Autodesk Inventor part; units mm, degrees
ref_plane "Work Plane1" through (0, 41.8, -12.9) normal (0, 0, 1) x (1, 0, 0)
ref_plane "YZ Plane" through (0, 0, 0) normal (1, 0, 0) x (0, 1, 0)
ref_plane "XZ Plane" through (0, 0, 0) normal (0, 1, 0) x (-1, 0, 0)
ref_plane "Work Plane1" through (0, 41.8, -12.9) normal (0, 0, 1) x (1, 0, 0)
sketch "Sketch1" plane through (0, 41.8, -12.9) normal (0, 0, 1) x (1, 0, 0)
  line L0 (3.85, 0.3752) -> (3.85, 4) construction
  line L1 (3.85, 4) -> (-2, 4) construction
  arc A0 (-2, 4) -> (-4, 2) centre (-2, 2) ccw construction
  line L2 (-4, 2) -> (-4, -3.85) construction
  line L3 (-4, -3.85) -> (-0.3752, -3.85) construction
  line L4 (-2, 4) -> (43.8, 4)
  line L5 (45.8, 2) -> (45.8, -43.8)
  line L6 (43.8, -45.8) -> (-2, -45.8)
  line L7 (-4, -43.8) -> (-4, 2)
  line L8 (40.3, -37.8) -> (40.3, -4)
  line L9 (37.8, -1.5) -> (4, -1.5)
  line L10 (1.5, -4) -> (1.5, -37.8)
  line L11 (4, -40.3) -> (37.8, -40.3)
  line L12 (37.8, -40.3) -> (40.3, -37.8)
  line L13 (4, -40.3) -> (1.5, -37.8)
  line L14 (4, -1.5) -> (1.5, -4)
  line L15 (40.3, -4) -> (37.8, -1.5)
  arc A1 (45.8, 2) -> (43.8, 4) centre (43.8, 2) ccw
  arc A2 (43.8, -45.8) -> (45.8, -43.8) centre (43.8, -43.8) ccw
  arc A3 (-4, -43.8) -> (-2, -45.8) centre (-2, -43.8) ccw
  arc A4 (-2, 4) -> (-4, 2) centre (-2, 2) ccw
  circle A5 centre (1, -1) radius 1.4
  circle A6 centre (40.8, -1) radius 1.4
  circle A7 centre (40.8, -40.8) radius 1.4
  circle A8 centre (1, -40.8) radius 1.4
  circle A9 centre (20.9, -20.9) radius 19.4 construction
  line L16 (3.85, -3.85) -> (3.85, -37.95)
  line L17 (3.85, -37.95) -> (37.95, -37.95)
  line L18 (37.95, -37.95) -> (37.95, -3.85)
  line L19 (37.95, -3.85) -> (3.85, -3.85)
  arc A10 (2.2654, -1.2094) -> (1.2094, -2.2654) centre (0.9, -0.9) ccw
  line L20 (2.2654, -1.2094) -> (3.85, 0.3752)
  line L21 (-0.3752, -3.85) -> (1.2094, -2.2654)
  point P0 (45.8, -45.8)
  point P1 (45.8, 4)
  point P2 (-4, -45.8)
  point P3 (40.3, -40.3)
  point P4 (40.3, -1.5)
  point P5 (1.5, -1.5)
  point P6 (1.5, -40.3)
  point P7 (40.8, -1)
  dimension "d55" = 2.8
  dimension "d34" = 49.8
  dimension "d35" = 49.8
  dimension "d36" = 5.5
  dimension "d37" = 2.5
  dimension "d38" = 2.5
  dimension "d39" = 2.5
  dimension "d40" = 2.5
  dimension "d41" = 2.5
  dimension "d42" = 2.5
  dimension "d43" = 2.5
  dimension "d44" = 2.5
  dimension "d45" = 2
  dimension "d46" = 5
  dimension "d47" = 5
  dimension "d48" = 5
  dimension "d49" = 5
  dimension "d51" = 5
  dimension "d52" = 0.5
  dimension "d53" = 5
  dimension "d54" = 5
  dimension "d56" = 2.8
  dimension "d57" = 2.8
  dimension "d58" = 2.8
  dimension "d90" = 7.85
extrude "Extrusion1" add sketch "Sketch1" along normal blind 7.7 contours L4 A1 L5 A2 L6 A3 L7 A4 | L12 L11 L13 L10 L14 L9 L15 L8 | A5 A10
fillet "Fillet1" radius 2 8 edges at (20.9, -4, -5.2) (45.2142, -3.4142, -5.2) (45.8, 20.9, -5.2) (45.2142, 45.2142, -5.2) (20.9, 45.8, -5.2) (-3.4142, 45.2142, -5.2) (-4, 20.9, -5.2) (-3.4142, -3.4142, -5.2)
sketch "Sketch3" plane through (0, 41.8, -5.2) normal (0, 0, 1) x (1, 0, 0)
  circle A0 centre (20.9, -20.9) radius 16.9 construction
  point P0 (0, -41.8)
sketch "Sketch4" plane through (0, 41.8, -5.2) normal (0, 0, 1) x (1, 0, 0)
  line L0 (37.95, -37.95) -> (37.95, -3.85)
  line L1 (37.95, -3.85) -> (3.85, -3.85)
  line L2 (3.85, -3.85) -> (3.85, -37.95)
  line L3 (3.85, -37.95) -> (37.95, -37.95)
  circle A0 centre (40.9, -0.9) radius 2.75
  circle A1 centre (0.9, -40.9) radius 2.75
  circle A2 centre (0.9, -0.9) radius 2.75
  circle A3 centre (40.9, -40.9) radius 2.75
  line L4 (34.3452, 2) -> (7.4548, 2)
  line L5 (43.8, -34.3452) -> (43.8, -7.4548)
  line L6 (7.4548, -43.8) -> (34.3452, -43.8)
  line L7 (-2, -7.4548) -> (-2, -34.3452)
  arc A4 (34.3452, 2) -> (36.4548, 2) centre (35.4, -0.1) ccw
  line L8 (43.8, 2) -> (36.4548, 2)
  line L9 (43.8, -5.3452) -> (43.8, 2)
  arc A5 (43.8, -5.3452) -> (43.8, -7.4548) centre (41.7, -6.4) ccw
  arc A6 (43.8, -34.3452) -> (43.8, -36.4548) centre (41.7, -35.4) ccw
  line L10 (43.8, -43.8) -> (43.8, -36.4548)
  line L11 (36.4548, -43.8) -> (43.8, -43.8)
  arc A7 (36.4548, -43.8) -> (34.3452, -43.8) centre (35.4, -41.7) ccw
  arc A8 (7.4548, -43.8) -> (5.3452, -43.8) centre (6.4, -41.7) ccw
  line L12 (-2, -43.8) -> (5.3452, -43.8)
  line L13 (-2, -36.4548) -> (-2, -43.8)
  arc A9 (-2, -36.4548) -> (-2, -34.3452) centre (0.1, -35.4) ccw
  arc A10 (-2, -7.4548) -> (-2, -5.3452) centre (0.1, -6.4) ccw
  line L14 (-2, 2) -> (-2, -5.3452)
  line L15 (5.3452, 2) -> (-2, 2)
  arc A11 (5.3452, 2) -> (7.4548, 2) centre (6.4, -0.1) ccw
hole "Hole2" at (40.9, 40.9, -5.2) at (40.9, 0.9, -5.2) at (0.9, 0.9, -5.2) at (0.9, 40.9, -5.2) direction (0, 0, -1) diameter 3.2 depth 12 tip angle 118 counterbore diameter 6 counterbore depth 3.1
chamfer "Chamfer2" distance 4.6 angle 45 2 edges at (3.85, 20.9, -12.9) (37.95, 20.9, -12.9)
sketch "Sketch9" plane through (37.95, 3.85, -5.2) normal (-1, 0, 0) x (0, 0, 1)
  line L0 (-7.7, 0) -> (-3.1, 0)
  line L1 (-3.1, 34.1) -> (-7.7, 34.1)
  line L2 (-3.1, 0) -> (-7.7, -4.6)
  line L3 (-7.7, 39.95) -> (-7.7, -5.85)
  line L4 (-3.1, 0) -> (3.4054, 0) construction
  line L5 (-7.7, -4.6) -> (-7.7, 0)
  line L6 (-3.1, 34.1) -> (-7.7, 38.7)
  line L7 (-3.1, 34.1) -> (3.4054, 34.1) construction
  line L8 (-7.7, 38.7) -> (-7.7, 34.1)
  line L9 (-7.7, 34.1) -> (-3.1, 34.1)
  point P0 (5.2, -3.85)
  point P1 (-7.7, -5.85)
  dimension "d91" = 135
  dimension "d92" = 135
extrude "Extrusion3" cut sketch "Sketch9" along normal up to surface (34.1 mm away)
sketch "Sketch14" plane through (0, 41.8, -5.2) normal (0, 0, 1) x (1, 0, 0)
  arc A0 (1.6681, -43.8) -> (-2, -40.1319) centre (0.9, -40.9) ccw construction
  line L0 (40.1319, -43.8) -> (1.6681, -43.8) construction
  arc A1 (43.8, -40.1319) -> (40.1319, -43.8) centre (40.9, -40.9) ccw construction
  line L1 (43.8, -1.6681) -> (43.8, -40.1319) construction
  arc A2 (40.1319, 2) -> (43.8, -1.6681) centre (40.9, -0.9) ccw construction
  line L2 (1.6681, 2) -> (40.1319, 2) construction
  arc A3 (-2, -1.6681) -> (1.6681, 2) centre (0.9, -0.9) ccw construction
  line L3 (-2, -40.1319) -> (-2, -1.6681) construction
  line L4 (3.85, -3.85) -> (37.95, -3.85) construction
  line L5 (37.95, -3.85) -> (37.95, -37.95) construction
  line L6 (37.95, -37.95) -> (3.85, -37.95) construction
  line L7 (3.85, -37.95) -> (3.85, -3.85) construction
  point P0 (0, -41.8)
  point P1 (6.4, -0.1)
  point P2 (0.1, -6.4)
  point P3 (0.1, -35.4)
  point P4 (6.4, -41.7)
  point P5 (35.4, -41.7)
  point P6 (41.7, -35.4)
  point P7 (41.7, -6.4)
  point P8 (35.4, -0.1)
hole "Hole6" [suppressed]
ref_plane "Work Plane5" through (20.9, -2, -12.9) normal (-1, 0, 0) x (0, 0, 1)
ref_plane "Work Plane6" through (-2, 20.9, -12.9) normal (0, -1, 0) x (1, 0, 0)
properties part number "10_Lid_1x1_v3"
Here's how the part is built. I have some questions about the finished solid (model axes, mm). A direction names the side the tool comes from. Give positions to 0.01 mm unless a question says otherwise; leave off trailing zeros. Order: outer loops, then holes, each group sorted by start corner. A loop starts at its lowest first (then second) coordinate and runs counter-clockwise, first axis right, second up. Notation, with made-up numbers: (64, 21.25) - (120, 21.25) arc R23 ccw to (120, 47.25) - close; hole circle Ø2 at (11.25, -8). An arc over 180 degrees is marked (long way). Answer as a JSON object with one key per item and string values. Group by question number.
Item 1: For P1, Ø3, axis at x = 20.5, y = 34.5, coming from the +Z side; P2, Ø0.9, axis at y = 26, z = -6, coming from the -X side; P3, Ø1.8, axis at x = 1.5, y = 0, coming from the +Z side; P4, Ø12, axis at x = 6.5, y = 21.5, coming from the -Z side, each with a flat end and sliding along its axis, tell me the tip position at first contact or that it passes through.
Item 2: If we section it at B-B on x = 30: Please give me the cut outline in (y, z).
Item 3: If we section it at D-D on y = 40.9: Please give me the cut outline in (x, z).
Item 4: If we mould it in two halves opening along X, with no side actions, what happens to faces 5 (the cylindrical face through (-3.43, 45.2, -10.09)), 6 (the flat face through (-1.4, 43.2, -5.2)), 7 (the flat face through (39, 37.95, -12))? For each: pulls with the +X half, pulls with the -X half, needs draft (parallel to the pull), parting line crosses it, or undercut.
Item 5: Please list where these lines run through material, in increasing order: probe 1 along X at (y, z) = (40.9, -11.85); probe 2 along Y at (x, z) = (0.9, -10.5); probe 3 along Y at (x, z) = (0.9, -7.3).
Item 6: Which directions (+Z, -Z, +X, -X, +Y, -Y) give clear straight access to the entire face, cutting with the end or side of a thin tool? Please do faces 1 (the cylindrical face through (45.23, 20.58, -5.8)), 2 (the cylindrical face through (0, 38.04, -6.77)), 3 (the flat face through (37.95, 21, -7)), 4 (the flat face through (3.85, 39, -12)).
Item 7: If we section it at A-A on z = -10.25: Please give me the cut outline in (x, y), and give its area (3 significant figures).
Result set:
{
 "1": {"P1": "through", "P2": "x = -3.85", "P3": "z = -8.3", "P4": "z = -11.65"},
 "2": {"outline": "(-4, -12.9) - (-0.75, -12.9) - (3.85, -8.3) - (3.85, -5.2) - (-2, -5.2) arc R2 ccw to (-4, -7.2) - close; (37.95, -8.3) - (42.55, -12.9) - (45.8, -12.9) - (45.8, -7.2) arc R2 ccw to (43.8, -5.2) - (37.95, -5.2) - close"},
 "3": {"outline": "(-4, -12.9) - (-0.7, -12.9) - (-0.7, -8.3) - (-2.1, -8.3) - (-2.1, -5.2) arc R2 ccw to (-4, -7.2) - close; (2.5, -12.9) - (3.85, -12.9) - (3.85, -11.25) - (37.95, -11.25) - (37.95, -12.9) - (39.3, -12.9) - (39.3, -8.3) - (37.9, -8.3) - (37.9, -5.2) - (3.9, -5.2) - (3.9, -8.3) - (2.5, -8.3) - close; (42.5, -12.9) - (45.8, -12.9) - (45.8, -7.2) arc R2 ccw to (43.9, -5.2) - (43.9, -8.3) - (42.5, -8.3) - close"},
 "4": {"face 5": "pulls with the -X half", "face 6": "needs draft", "face 7": "undercut"},
 "5": {"probe 1": "-4 to -0.7, 2.5 to 3.85, 37.95 to 39.3, 42.5 to 45.8", "probe 2": "-4 to -0.7, 2.5 to 39.3, 42.5 to 45.8", "probe 3": "-4 to -2.1, 3.9 to 37.9, 43.9 to 45.8"},
 "6": {"face 1": "+Z, +X, +Y, -Y", "face 2": "+Z", "face 3": "+Z, -Z", "face 4": "-Z"},
 "7": {"outline": "(-4, -2) arc R2 ccw to (-2, -4) - (43.8, -4) arc R2 ccw to (45.8, -2) - (45.8, 43.8) arc R2 ccw to (43.8, 45.8) - (-2, 45.8) arc R2 ccw to (-4, 43.8) - close; hole circle Ø3.2 at (0.9, 0.9); hole circle Ø3.2 at (0.9, 40.9); hole (1.9, 3.85) - (3.85, 3.85) - (3.85, 1.9) - (37.95, 1.9) - (37.95, 3.85) - (39.9, 3.85) - (39.9, 37.95) - (37.95, 37.95) - (37.95, 39.9) - (3.85, 39.9) - (3.85, 37.95) - (1.9, 37.95) - close; hole circle Ø3.2 at (40.9, 0.9); hole circle Ø3.2 at (40.9, 40.9)", "area": "1,020 mm²"}
}
